from build123d import *

# Parameters (mm, degrees)
F0_R     = 14
F0_R_2   = 9
F0_R_3   = 7.5
F1_DEPTH = 20
F2_R     = 14
F2_R_2   = 6.5
F2_R_3   = 4.75
F3_DEPTH = 40
F4_R     = 5
F5_R     = 3


with BuildPart() as f1:
    # F0 (on Top) → F1 (new body)
    with BuildSketch(Plane.XY):
        Circle(F0_R)
        Circle(F0_R_2, mode=Mode.SUBTRACT)
        Circle(F0_R_2)
        Circle(F0_R_3, mode=Mode.SUBTRACT)
        Circle(F0_R_3)
    extrude(amount=F1_DEPTH)

    # F2 (on face) → F3 (join)
    with BuildSketch(Plane.XY.offset(20)):
        Circle(F2_R)
        Circle(F2_R_2, mode=Mode.SUBTRACT)
        Circle(F2_R_3)
    extrude(amount=F3_DEPTH)

    # F4
    f4_edges = [f1.edges().sort_by_distance(p)[0] for p in [
        (-14, 0, 0),
    ]]
    fillet(f4_edges, radius=F4_R)

    # F5
    f5_edges = [f1.edges().sort_by_distance(p)[0] for p in [
        (-14, 0, 60),
    ]]
    fillet(f5_edges, radius=F5_R)


solid = f1.part
For this review, take the finished solid that the model builds, in its own axes (mm). A direction names the side the tool comes from. Give positions to 0.01 mm unless a question says otherwise; leave off trailing zeros. Order: outer loops, then holes, each group sorted by start corner. A loop starts at its lowest first (then second) coordinate and runs counter-clockwise, first axis right, second up. Notation, with made-up numbers: (14, -36) - (30, -36) arc R32 ccw to (30, 2) - close; hole circle Ø10 at (88, 80.5). An arc over 180 degrees is marked (long way). Answer as a JSON object with one key per item and string values. Group by question number.
Item 1: Clearance check with flat-ended pins moving along their axes: pin 1 Ø5 at (x, z) = (6.5, 12.5) entering from -Y; pin 2 Ø3 at (x, z) = (-10.5, 21.5) entering from +Y; pin 3 Ø4 at (y, z) = (-3, 28) entering from +X. State where each tip first meets the part, or that it passes through.
Item 2: Machinability: for faces 5 (the cylindrical face through (-5.158, -3.955, 39.72)), 6 (the flat face through (5, -5, 60)), which of the approach directions +Z, -Z, +X, -X, +Y, -Y give a long, thin tool a straight path to every point of the face, cutting with its end or side? Answer none if there is none.
Item 3: Take a section at A-A on z = 24. Give the boundary of the cut face in (x, y).
Item 4: Draft analysis for pull direction Y (two halves, no side actions). For faces 1 (the flat face through (0, -5, 20)), 2 (the flat face through (0, 0, 0)), 3 (the cylindrical face through (2.192, -4.214, 39.72)), 4 (the cylindrical face through (12.932, -5.362, 30.636)), state which applies: pulls with the +Y half, pulls with the -Y half, needs draft (parallel to the pull), parting line crosses it, or undercut.
Item 5: Wall thickness on line 1 along Y through (x, z) = (0, 36); line 2 along Y through (x, z) = (-2.5, 36.5); line 3 along X through (y, z) = (0.5, 55): over which ranges is each line inside the solid? List them lowest first.
Item 6: Take a section at D-D on z = 14. Give the boundary of the cut face in (x, y), and give its area (3 significant figures).
Item 7: Take a section at B-B on x = 0. Give the boundary of the cut face in (y, z).
Reported:
{
 "1": {"pin 1": "y = -13.42", "pin 2": "y = 10.72", "pin 3": "x = 13.96"},
 "2": {"face 5": "+Z", "face 6": "+Z, +X, -X, +Y, -Y"},
 "3": {"outline": "circle Ø28 at (0, 0); circle Ø9.5 at (0, 0); hole circle Ø13 at (0, 0)"},
 "4": {"face 1": "undercut", "face 2": "needs draft", "face 3": "undercut", "face 4": "parting line crosses it"},
 "5": {"line 1": "-14 to -6.5, -4.75 to 4.75, 6.5 to 14", "line 2": "-13.77 to -6, -4.04 to 4.04, 6 to 13.77", "line 3": "-13.99 to -6.48, -4.72 to 4.72, 6.48 to 13.99"},
 "6": {"outline": "circle Ø28 at (0, 0)", "area": "616 mm^2"},
 "7": {"outline": "(-14, 5) arc R5 ccw to (-9, 0) - (9, 0) arc R5 ccw to (14, 5) - (14, 57) arc R3 ccw to (11, 60) - (6.5, 60) - (6.5, 20) - (4.75, 20) - (4.75, 60) - (-4.75, 60) - (-4.75, 20) - (-6.5, 20) - (-6.5, 60) - (-11, 60) arc R3 ccw to (-14, 57) - close"}
}
